from build123d import *

# Parameters (mm, degrees)
SKETCH1_R           = 6.725
SKETCH1_R_2         = 3.05
BOSS_EXTRUDE1_DEPTH = 4.5
SKETCH3_R           = 3.05
BOSS_EXTRUDE3_DEPTH = 1
BOSS_EXTRUDE4_DEPTH = 3
SKETCH5_R           = 8.225
SKETCH5_R_2         = 6.725
BOSS_EXTRUDE5_DEPTH = 9
FILLET1_R           = 0.2
CUT_EXTRUDE1_REACH  = 14.867
SKETCH6_R           = 1.25
SKETCH7_W           = 2
SKETCH7_H           = 1
CUT_EXTRUDE2_DEPTH  = 3.5
CHAMFER1_SIZE       = 0.5


# Read off the part's stored shape, not the designer's step: Boss-Extrude2
with BuildPart() as part:
    # Sketch1 → Boss-Extrude1 (new body)
    with BuildSketch(Plane.XY):
        Circle(SKETCH1_R)
        Circle(SKETCH1_R_2, mode=Mode.SUBTRACT)
    extrude(amount=BOSS_EXTRUDE1_DEPTH)

    # Boss-Extrude2 outline → Boss-Extrude2 (revolve)
    with BuildSketch(Plane.XZ):
        with BuildLine():
            Line((6.725000003, -3.25921624), (6.725, 1e-09))
            Line((6.725, 1e-09), (3.599999993, 4e-09))
            ThreePointArc((3.599999993, 4e-09), (5.413596666, -1.388851743), (6.725000003, -3.25921624))
        make_face()
    revolve(axis=Axis((0, 0, 0), (0, 0, 1)))

    # Sketch3 → Boss-Extrude3 (add)
    with BuildSketch(Plane(origin=(0, 0, 0), x_dir=(-1, 0, 0), z_dir=(0, 0, -1))):
        Circle(SKETCH3_R)
    extrude(amount=-BOSS_EXTRUDE3_DEPTH)

    # Sketch4 → Boss-Extrude4 (add)
    with BuildSketch(Plane(origin=(0, 0, 0), x_dir=(-1, 0, 0), z_dir=(0, 0, -1))):
        Polygon((0, -2.944486373), (2.55, -1.472243186), (2.55, 1.472243186), (0, 2.944486373), (-2.55, 1.472243186), (-2.55, -1.472243186), align=None)
    extrude(amount=BOSS_EXTRUDE4_DEPTH)

    # Sketch5 → Boss-Extrude5 (add)
    with BuildSketch(Plane.XY.offset(4.5)):
        Circle(SKETCH5_R)
        Circle(SKETCH5_R_2, mode=Mode.SUBTRACT)
    extrude(amount=-BOSS_EXTRUDE5_DEPTH)

    # Fillet1
    fillet1_edges = [part.edges().sort_by_distance(p)[0] for p in [
        (1.275, -2.20836478, 0),
        (2.55, -1.472243186, -1.5),
        (-1.275, -2.20836478, 0),
        (0, -2.944486373, -1.5),
        (-2.55, 0, 0),
        (-2.55, -1.472243186, -1.5),
        (-1.275, 2.20836478, 0),
        (-2.55, 1.472243186, -1.5),
        (1.275, 2.20836478, 0),
        (0, 2.944486373, -1.5),
        (2.55, 0, 0),
        (2.55, 1.472243186, -1.5),
        (1.275, -2.20836478, -3),
        (-1.275, -2.20836478, -3),
        (-2.55, 0, -3),
        (-1.275, 2.20836478, -3),
        (1.275, 2.20836478, -3),
        (2.55, 0, -3),
        (-8.225, 0, -4.5),
        (-6.725, 0, -4.5),
        (-3.599999993, 0, 4e-09),
    ]]
    fillet(fillet1_edges, radius=FILLET1_R)

    # Sketch6 → Cut-Extrude1 (cut, up to next)
    with BuildSketch(Plane.XY.offset(1), mode=Mode.PRIVATE) as cut_extrude1_sk1:
        Circle(SKETCH6_R)
    cut_extrude1_tool1 = extrude(cut_extrude1_sk1.sketch, amount=-CUT_EXTRUDE1_REACH, mode=Mode.PRIVATE) & part.part
    add(cut_extrude1_tool1.solids().sort_by_distance((0, 0, 1))[0], mode=Mode.SUBTRACT)

    # Sketch7 → Cut-Extrude2 (cut)
    with BuildSketch(Plane.XY.offset(4.5)):
        with Locations((0, 3.381405907)):
            Rectangle(SKETCH7_W, SKETCH7_H)
        with Locations((0, -3.381405907)):
            Rectangle(SKETCH7_W, SKETCH7_H)
    extrude(amount=-CUT_EXTRUDE2_DEPTH, mode=Mode.SUBTRACT)

    # Chamfer1
    chamfer1_edges = [part.edges().sort_by_distance(p)[0] for p in [
        (-3.05, 0, 4.5),
        (3.05, 0, 4.5),
        (1, 3.381405907, 4.5),
        (0, 3.881405907, 4.5),
        (-1, 3.381405907, 4.5),
        (1, -3.381405907, 4.5),
        (-1, -3.381405907, 4.5),
        (0, -3.881405907, 4.5),
        (-8.225, 0, 4.5),
    ]]
    chamfer(chamfer1_edges, length=CHAMFER1_SIZE)


solid = part.part
CAD build for the part. Positions are in the model's coordinates, mm. A direction names the side the tool comes from. Give positions to 0.01 mm unless a question says otherwise; leave off trailing zeros. Write each loop counter-clockwise with the first axis right and the second up, starting at its lowest first coordinate (ties: lowest second). Pieces come first, ordered by that corner, then holes. Notation, with made-up numbers: M 0.25,25.25 L 57.25,25.25 A26 ccw 57.25,59.25 Z; hole C 75,39.25 d11. An arc over 180 degrees is marked long. Put each result on its own line as item: value. Start each with the question number.
(1) Band-saw the part on A-A, the plane z = -4. Write the cut outline in (x, y) (3 decimals), and give its area (3 significant figures).
(2) Which spindle directions (+Z, -Z, +X, -X, +Y, -Y) get a long thin tool onto all of the face, cutting with end or side? Do faces 3 (the face through (-1, 3.4, 2.5)), 4 (the face through (2.55, 0, -1)). Say none if no direction does.
(3) Mould opens along Y. For faces 1 (the face through (-1.8, -3.3, 4.5)), 2 (the face through (1.4, 0.1, 1)) say: +Y half, -Y half, draft (parallel to the pull), parting line (faces both ways), or undercut.
(4) Band-saw the part on B-B, the plane z = 0.5. Write the cut outline in (x, y) (3 decimals).
(5) Probe L1, parallel to Y at x = 0, z = -3.8 (3 decimals); L2, parallel to Y at x = 1.5, z = -1; L3, parallel to Y at x = -0.75, z = 2.5. List the from-to ranges inside material, lowest first.
(6) Flat gauge pins, fed straight in: pin 1 Ø5.5 at (x, y) = (-0.5, -0.5) entering from -Z; pin 2 Ø5 at (x, z) = (-2.5, 3.5) entering from +Y (3 decimals); pin 3 Ø1.5 at (y, z) = (-1.5, 0) entering from +X; pin 4 Ø1.5 at (x, y) = (-2, 1) entering from +Z. Where does each tip first touch, or does it go through?
Response values:
1. outline: C 0,0 d16.45; hole C 0,0 d13.45
1. area: 70.5 mm2
2. face 3: +Z
2. face 4: -Z
3. face 1: draft
3. face 2: undercut
4. outline: C 0,0 d16.45; hole C 0,0 d2.5
5. L1: y = -8.225 to -6.725, 6.725 to 8.225
5. L2: y = -8.09 to -4.78, -2.08 to 2.08, 4.78 to 8.09
5. L3: y = -8.19 to -3.88, 3.88 to 8.19
6. pin 1: stops at z = -3
6. pin 2: stops at y = 8.225
6. pin 3: stops at x = 8.19
6. pin 4: stops at z = 1
